```python
from build123d import *

# Parameters (mm, degrees)
ESQUISSE1_W             = 100
ESQUISSE1_H             = 82
BOSS_EXTRU_1_DEPTH      = 6
ESQUISSE2_R             = 1.75
ENL_V_MAT_EXTRU_1_DEPTH = 6
ESQUISSE3_R             = 1.75
ENL_V_MAT_EXTRU_2_DEPTH = 6


with BuildPart() as part:
    # Esquisse1 → Boss.-Extru.1 (new body)
    with BuildSketch(Plane.XY):
        Rectangle(ESQUISSE1_W, ESQUISSE1_H)
    extrude(amount=BOSS_EXTRU_1_DEPTH)

    # Esquisse2 → Enlèv. mat.-Extru.1 (cut)
    with BuildSketch(Plane.XY):
        with Locations(Location((-25, -38, 0), (0, 0, 180))):
            Circle(ESQUISSE2_R)
        with Locations(Location((25, -38, 0), (0, 0, 180))):
            Circle(ESQUISSE2_R)
        with Locations(Location((-25, 38, 0), (0, 0, 180))):
            Circle(ESQUISSE2_R)
        with Locations(Location((25, 38, 0), (0, 0, 180))):
            Circle(ESQUISSE2_R)
    extrude(amount=ENL_V_MAT_EXTRU_1_DEPTH, mode=Mode.SUBTRACT)

    # Esquisse3 → Enlèv. mat.-Extru.2 (cut)
    with BuildSketch(Plane.XY):
        with Locations(Location((47, 0, 0), (0, 0, 180))):
            Circle(ESQUISSE3_R)
    enl_v_mat_extru_2 = extrude(amount=ENL_V_MAT_EXTRU_2_DEPTH, mode=Mode.SUBTRACT)

    # Symétrie1: Enlèv. mat.-Extru.2 across plane
    add(enl_v_mat_extru_2.mirror(Plane(origin=(0, 0, 0), x_dir=(0, 0, 1), z_dir=(1, 0, 0))), mode=Mode.SUBTRACT)


solid = part.part
```
Model file for the job. Use its own axes, mm. Round coordinates to 2 decimals unless told otherwise and drop trailing zeros. Order: outer loops, then holes, each group sorted by start corner. A loop starts at its lowest first (then second) coordinate and runs counter-clockwise, first axis right, second up. Notation, with made-up numbers: M -18,-31.75 L -13,-31.75 A9 cw -13,-15.75 Z; hole C -7,-17 d7. An arc over 180 degrees is marked long. Use CSV: the item, a comma, the result in double quotes.
Item 1: Pull direction Y, two halves, no side cores. Call faces 1 (the face through (-1, 41, 3)), 2 (the face through (-1, -41, 3)), 3 (the face through (-45.383, 0.67, 2.958)), 4 (the face through (-1, 1, 6)): released by +Y, released by -Y, zero draft, split by the parting line, or undercut.
Worked answers:
face 1,"released by +Y"
face 2,"released by -Y"
face 3,"undercut"
face 4,"zero draft"
Item 2: Saw through at B-B (y = 38). List the corners of the cut face in (x, z).
Worked answers:
outline,"M -50,0 L -26.75,0 L -26.75,6 L -50,6 Z; M -23.25,0 L 23.25,0 L 23.25,6 L -23.25,6 Z; M 26.75,0 L 50,0 L 50,6 L 26.75,6 Z"
Item 3: Saw through at C-C (x = 25). List the corners of the cut face in (y, z), plus the area to 3 significant figures.
Worked answers:
outline,"M -41,0 L -39.75,0 L -39.75,6 L -41,6 Z; M -36.25,0 L 36.25,0 L 36.25,6 L -36.25,6 Z; M 39.75,0 L 41,0 L 41,6 L 39.75,6 Z"
area,"450 mm²"
Item 4: Saw through at A-A (x = -47). List the corners of the cut face in (y, z), plus the area to 3 significant figures.
Worked answers:
outline,"M -41,0 L -1.75,0 L -1.75,6 L -41,6 Z; M 1.75,0 L 41,0 L 41,6 L 1.75,6 Z"
area,"471 mm²"
Item 5: Probe probe 1 along X at (y, z) = (-38, 2.55); probe 2 along Y at (x, z) = (25, 2.2); probe 3 along Y at (x, z) = (-47, 4.15). List the from-to ranges inside material, lowest first.
Worked answers:
probe 1,"-50 to -26.75, -23.25 to 23.25, 26.75 to 50"
probe 2,"-41 to -39.75, -36.25 to 36.25, 39.75 to 41"
probe 3,"-41 to -1.75, 1.75 to 41"
